Design review of the part shown in the three views and the two pictorial views. Dimensions are in mm from the part's minimum x, y and z. Round coordinates to 2 decimals unless told otherwise and drop trailing zeros. Order: outer loops, then holes, each group sorted by start corner. A loop starts at its lowest first (then second) coordinate and runs counter-clockwise, first axis right, second up.
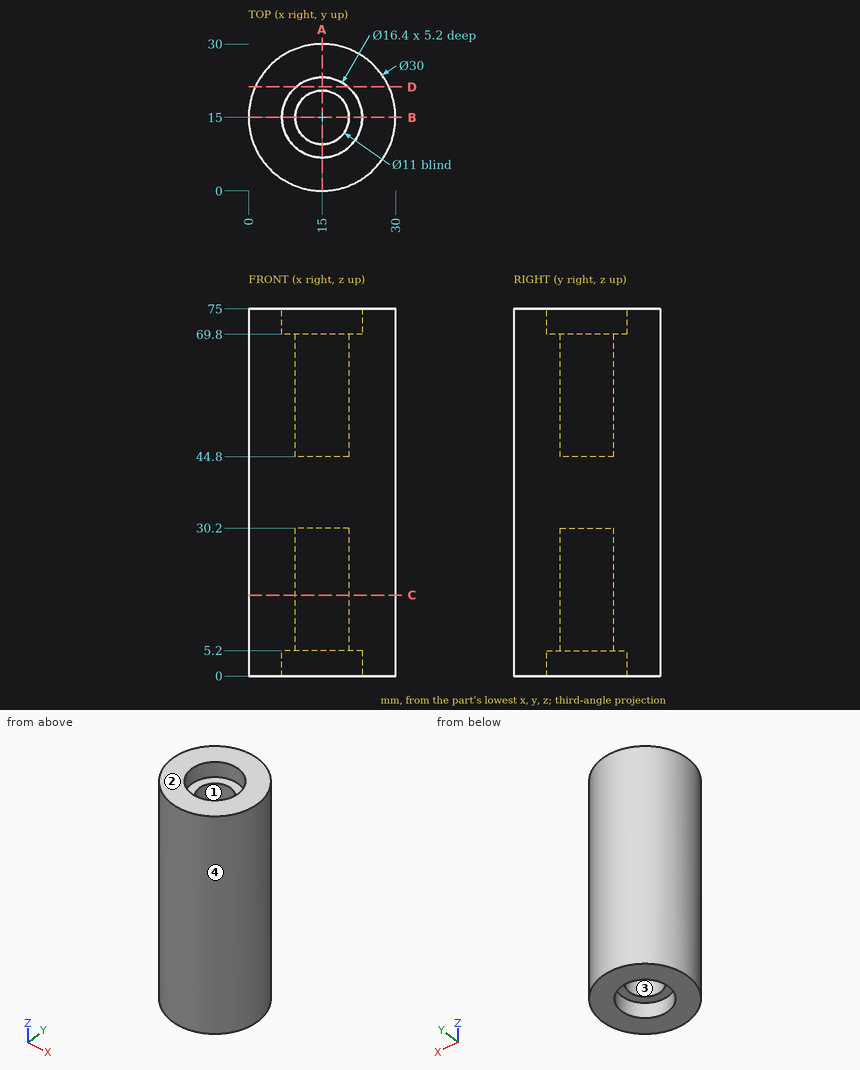
(1) Draft analysis for pull direction Y (two halves, no side actions). For the marked faces 1, 2, 3 and 4, state which applies: pulls with the +Y half, pulls with the -Y half, needs draft (parallel to the pull), parting line crosses it, or undercut.
(2) Add section A-A on x = 15. Give the boundary of the cut face in (y, z).
(3) Add section D-D on y = 21.25. Give the boundary of the cut face in (x, z), plus the area to 3 significant figures.
(4) Wall thickness on L1, parallel to Y at x = 15, z = 62.25; L2, parallel to Y at x = 15, z = 70.95; L3, parallel to Z at x = 15.5, y = 22: over which ranges is each line inside the solid? List them lowest first.
(5) Clearance check with flat-ended pins moving along their axes: P1, Ø4, axis at y = 10, z = 9, coming from the +X side; P2, Ø14.5, axis at x = 15, y = 15, coming from the -Z side; P3, Ø6, axis at x = 10, z = 62, coming from the -Y side. State where each tip first meets the part, or that it passes through.
(6) Add section C-C on z = 16.5. Give the boundary of the cut face in (x, y), plus the area to 3 significant figures.
Here are the results:
1. face 1: undercut
1. face 2: needs draft
1. face 3: undercut
1. face 4: parting line crosses it
2. outline: (0, 0) - (6.8, 0) - (6.8, 5.2) - (9.5, 5.2) - (9.5, 30.2) - (20.5, 30.2) - (20.5, 5.2) - (23.2, 5.2) - (23.2, 0) - (30, 0) - (30, 75) - (23.2, 75) - (23.2, 69.8) - (20.5, 69.8) - (20.5, 44.8) - (9.5, 44.8) - (9.5, 69.8) - (6.8, 69.8) - (6.8, 75) - (0, 75) - close
3. outline: (1.36, 0) - (9.69, 0) - (9.69, 5.2) - (20.31, 5.2) - (20.31, 0) - (28.64, 0) - (28.64, 75) - (20.31, 75) - (20.31, 69.8) - (9.69, 69.8) - (9.69, 75) - (1.36, 75) - close
3. area: 1,930 mm2
4. L1: y = 0 to 9.5, 20.5 to 30
4. L2: y = 0 to 6.8, 23.2 to 30
4. L3: z = 5.2 to 69.8
5. P1: stops at x = 29.7
5. P2: stops at z = 5.2
5. P3: stops at y = 0.13
6. outline: circle Ø30 at (15, 15); hole circle Ø11 at (15, 15)
6. area: 612 mm2
